Source: three-view drawing plus pictorial views. Frame: mm from the lowest corner of the part. Coordinates: 2 decimals unless noted, no trailing zeros. Write each question's results on one line, items separated by ' | '. Start each with the question number.
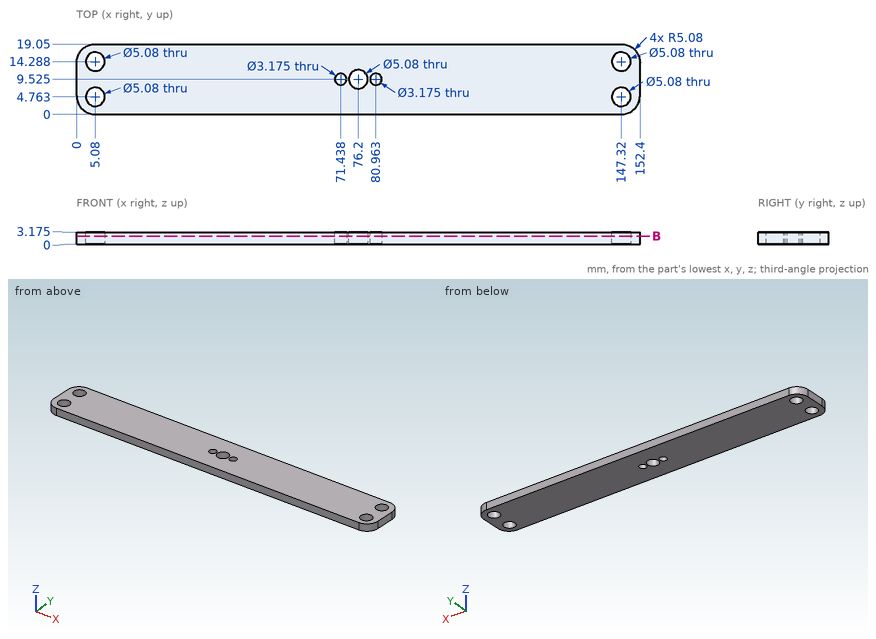
Item 1: Contact query for a flat-ended pin moving along its axis: P1, Ø4, axis at x = 71.44, y = 9.53, coming from the +Z side (1 decimal). Output: stop coordinate, or through.
Item 2: Ray query, L1, parallel to X at y = 9.75, z = 2.2 (1 decimal); L2, parallel to Y at x = 5.08, z = 1.8; L3, parallel to X at y = 4, z = 2.25 (1 decimal). Return the intervals inside material, ascending. Write a range as [from, to].
Item 3: Section B-B, the plane z = 2.2. Count the separate pieces of the cut face and the enclosed holes in it, plus the area to 3 significant figures.
Solutions:
1) P1: stops at z = 3.2
2) L1: x = [0, 69.9], [73, 73.7], [78.7, 79.4], [82.5, 152.4] | L2: y = [0, 2.22], [7.3, 11.75], [16.83, 19.05] | L3: x = [0.1, 2.7], [7.5, 144.9], [149.7, 152.3]
3) separate pieces: 1 | enclosed holes: 7 | area: 2,760 mm²
